Build history of the part. All positions in model axes, mm. A direction names the side the tool comes from. Coordinates: 2 decimals unless noted, no trailing zeros. Loops run counter-clockwise (first coordinate to the right, second up) from the corner with the lowest first, then second, coordinate; pieces in that order, holes last. Notation, with made-up numbers: M 82,-21 L 92,-21 A12 ccw 92,-15 Z; hole C -38.75,42 d8. An arc over 180 degrees is marked long. Write each question's results on one line, items separated by ' | '. Start each with the question number.
from build123d import *

# Parameters (mm, degrees)
SKETCH_1_W          = 121
SKETCH_1_H          = 146
EXTRUDE_1_DEPTH     = 3
FILLET_1_R          = 10
SKETCH_2_R          = 1.6
CUT_EXTRUDE_1_DEPTH = 4
SKETCH_3_W          = 81
SKETCH_3_H          = 20
CUT_EXTRUDE_2_DEPTH = 4


with BuildPart() as part:
    # Sketch 1 → ﾎﾞｽ - 押し出し1 (new body)
    with BuildSketch(Plane.XY):
        with Locations((60.5, 73)):
            Rectangle(SKETCH_1_W, SKETCH_1_H)
    extrude(amount=EXTRUDE_1_DEPTH)

    # ﾌｨﾚｯﾄ1
    fillet_1_edges = [part.edges().sort_by_distance(p)[0] for p in [
        (0, 146, 1.5),
        (121, 146, 1.5),
        (121, 0, 1.5),
        (0, 0, 1.5),
    ]]
    fillet(fillet_1_edges, radius=FILLET_1_R)

    # ｽｹｯﾁ2 → ｶｯﾄ - 押し出し1 (cut, through all)
    with BuildSketch(Plane.XY.offset(3)):
        with Locations((10, 136)):
            Circle(SKETCH_2_R)
        with Locations((10, 70.035204196)):
            Circle(SKETCH_2_R)
        with Locations((111, 136)):
            Circle(SKETCH_2_R)
        with Locations((111, 70)):
            Circle(SKETCH_2_R)
        with Locations((111, 10)):
            Circle(SKETCH_2_R)
        with Locations((10, 10)):
            Circle(SKETCH_2_R)
    extrude(amount=-CUT_EXTRUDE_1_DEPTH, mode=Mode.SUBTRACT)

    # ｽｹｯﾁ3 → ｶｯﾄ - 押し出し2 (cut, through all)
    with BuildSketch(Plane.XY.offset(3)):
        with Locations((60.5, 40)):
            Rectangle(SKETCH_3_W, SKETCH_3_H)
    extrude(amount=-CUT_EXTRUDE_2_DEPTH, mode=Mode.SUBTRACT)


solid = part.part
1. Mould opens along X. For faces 1 (the cylindrical face through (118.15, 142.99, 1.52)), 2 (the cylindrical face through (8.4, 10.07, 1.52)), 3 (the cylindrical face through (2.85, 142.99, 1.52)) say: +X half, -X half, draft (parallel to the pull), parting line (faces both ways), or undercut.
2. Band-saw the part on A-A, the plane x = 73.5. List the corners of the cut face in (y, z), plus the area to 3 significant figures.
3. Which spindle directions (+Z, -Z, +X, -X, +Y, -Y) get a long thin tool onto all of the face, cutting with end or side? Do faces 4 (the flat face through (60, 30, 2)), 5 (the flat face through (60, 146, 1)). Say none if no direction does.
4. Wall check: line 1 along Y through (x, z) = (111, 1); line 2 along X through (y, z) = (136, 0.9); line 3 along Y through (x, z) = (89, 1.1). Give the ranges that are in metal, low to high.
5. Pin check, flat tip, straight feed: pin 1 (1.9 mm diameter, centred on x = 111, y = 136, fed in from -Z). Stop position of the tip, or through.
Checked values:
1) face 1: +X half | face 2: undercut | face 3: -X half
2) outline: M 0,0 L 30,0 L 30,3 L 0,3 Z; M 50,0 L 146,0 L 146,3 L 50,3 Z | area: 378 mm²
3) face 4: +Z, -Z | face 5: +Z, -Z, +X, -X, +Y
4) line 1: 0 to 8.4, 11.6 to 68.4, 71.6 to 134.4, 137.6 to 146 | line 2: 0 to 8.4, 11.6 to 109.4, 112.6 to 121 | line 3: 0 to 30, 50 to 146
5) pin 1: through
